The listing builds one solid part. Answer for the finished solid, in the listing's coordinates (mm). A direction names the side the tool comes from. Coordinates: 2 decimals unless noted, no trailing zeros. Write each loop counter-clockwise with the first axis right and the second up, starting at its lowest first coordinate (ties: lowest second). Pieces come first, ordered by that corner, then holes.
Autodesk Inventor part; units mm, degrees
ref_plane "YZ Plane" through (0, 0, 0) normal (1, 0, 0) x (0, 1, 0)
ref_plane "XZ Plane" through (0, 0, 0) normal (0, 1, 0) x (-1, 0, 0)
ref_plane "XY Plane" through (0, 0, 0) normal (0, 0, 1) x (1, 0, 0)
sketch "Sketch1" plane through (0, 0, 0) normal (0, 1, 0) x (-1, 0, 0)
  line L0 (4, 7.5) -> (-4, 7.5)
  line L1 (-4, 7.5) -> (-4, -7.5)
  line L2 (-4, -7.5) -> (4, -7.5)
  line L3 (4, -7.5) -> (4, 7.5)
  line L4 (4, 7.5) -> (-4, -7.5) construction
  line L5 (-4, 7.5) -> (4, -7.5) construction
  point P0 (0, 0)
  dimension "d0" = 8
  dimension "d1" = 15
extrude "Extrusion1" add sketch "Sketch1" along normal blind 10
sketch "Sketch2" plane through (0, 10, 0) normal (0, 1, 0) x (1, 0, 0)
  line L0 (4, 7.5) -> (-4, 7.5)
  line L1 (-1.5, -7.5) -> (1.5, -7.5)
  line L2 (1.5, -7.5) -> (1.5, 7.5)
  line L3 (1.5, 7.5) -> (-1.5, 7.5)
  line L4 (-1.5, 7.5) -> (-1.5, -7.5)
  line L5 (-1.5, -7.5) -> (1.5, 7.5) construction
  line L6 (1.5, -7.5) -> (-1.5, 7.5) construction
  point P0 (0, 0)
  dimension "d4" = 3
extrude "Extrusion2" cut sketch "Sketch2" against normal blind 5
thicken "Thicken1" operation add thickness 2 both sides no extend neighbours yes toward (0, 1, 0) faces at (2.3333, 10, -2.5)
thicken "Thicken2" operation add thickness 2 both sides no extend neighbours yes toward (0, 1, 0) faces at (-3.1667, 10, -2.5)
thicken "Thicken3" operation add thickness 1 both sides no extend neighbours yes toward (0, 1, 0) faces at (-3.1667, 12, -2.5)
thicken "Thicken4" operation add thickness 1 both sides no extend neighbours yes toward (0, 1, 0) faces at (3.1667, 12, 2.5)
fillet "Fillet1" radius 1 10 edges at (4, 6.5, 7.5) (4, 6.5, -7.5) (-4, 6.5, 7.5) (-4, 6.5, -7.5) (4, 13, 0) (-4, 13, 0) (2.75, 13, -7.5) (2.75, 13, 7.5) (-2.75, 13, 7.5) (-2.75, 13, -7.5)
sketch "Sketch3" plane through (0, 0, 0) normal (0, -1, 0) x (1, 0, 0)
  arc A0 (-3, 7.5) -> (-4, 6.5) centre (-3, 6.5) ccw construction
  line L0 (-4, -6.5) -> (-4, 6.5) construction
  arc A1 (-4, -6.5) -> (-3, -7.5) centre (-3, -6.5) ccw construction
  line L1 (3, -7.5) -> (-3, -7.5) construction
  arc A2 (3, -7.5) -> (4, -6.5) centre (3, -6.5) ccw construction
  line L2 (4, 6.5) -> (4, -6.5) construction
  arc A3 (4, 6.5) -> (3, 7.5) centre (3, 6.5) ccw construction
  line L3 (-3, 7.5) -> (3, 7.5) construction
  point P0 (0, 0)
  point P1 (0, 0)
hole "Hole1" at (0, 0, 0) direction (0, 1, 0) diameter 2.85 depth 5
thicken "Thicken7" operation add thickness 0.1 both sides no extend neighbours yes toward (-1, 0, 0) faces at (1.5, 7.6667, -2.1667)
thicken "Thicken8" operation add thickness 0.1 both sides no extend neighbours yes toward (1, 0, 0) faces at (-1.5, 7.6667, 2.1667)
properties part number "zoffset"
(1) Section D-D, the plane y = 3.5 is taken. Write down the section's boundary in (x, z) (3 decimals), plus the area to 3 significant figures.
(2) This flat-tipped pin is pushed along its axis until it touches: pin 1 (0.8 mm diameter, centred on x = -0.5, z = -3.5, fed in from +Y). Where does it stop, or does it pass through?
(3) Find the intervals of material crossed by probe 1 along X at (y, z) = (10.25, -1.5); probe 2 along Z at (x, y) = (0, 2.75) (3 decimals); probe 3 along Y at (x, z) = (1, -4), in increasing order.
(4) Section B-B, the plane x = 0 is taken. Write down the section's boundary in (y, z) (3 decimals).
(5) Which of the six approach directions +Z, -Z, +X, -X, +Y, -Y give full straight-line access (tool end or side, diameter ignored) to faces 5 (the cylindrical face through (-2.211, 12.699, 7.215)), 6 (the flat face through (-1.4, 9, 0))?
(6) Section A-A, the plane y = 10.25 is taken. Write down the section's boundary in (x, z).
(7) Section C-C, the plane z = 0 is taken. Write down the section's boundary in (x, y) (3 decimals).
(8) For a pull along Z with two mould halves and no side action, classify faces 1 (the cylindrical face through (3.699, 6.084, 7.215)), 2 (the flat face through (0, 4.8, -7.5)), 3 (the flat face through (2, 13, 0)), 4 (the cylindrical face through (0.87, 2.54, 1.13)) as pulls with the +Z half, pulls with the -Z half, needs draft (parallel to the pull), parting line crosses it, or undercut.
Solution:
1. outline: (-4, -6.5) arc R1 ccw to (-3, -7.5) - (3, -7.5) arc R1 ccw to (4, -6.5) - (4, 6.5) arc R1 ccw to (3, 7.5) - (-3, 7.5) arc R1 ccw to (-4, 6.5) - close; hole circle Ø2.85 at (0, 0)
1. area: 113 mm2
2. pin 1: stops at y = 5
3. probe 1: x = -4 to -1.4, 1.4 to 4
3. probe 2: z = -7.5 to -1.425, 1.425 to 7.5
3. probe 3: y = 0 to 5
4. outline: (0, -7.5) - (5, -7.5) - (5, -1.425) - (0, -1.425) - close; (0, 1.425) - (5, 1.425) - (5, 7.5) - (0, 7.5) - close
5. face 5: +Z, +X, -X, +Y
5. face 6: +Z, -Z, +Y
6. outline: (-4, -6.5) arc R1 ccw to (-3, -7.5) - (-1.4, -7.5) - (-1.4, 7.5) - (-3, 7.5) arc R1 ccw to (-4, 6.5) - close; (1.4, -7.5) - (3, -7.5) arc R1 ccw to (4, -6.5) - (4, 6.5) arc R1 ccw to (3, 7.5) - (1.4, 7.5) - close
7. outline: (-4, 0) - (-1.425, 0) - (-1.425, 5) - (-1.4, 5) - (-1.4, 13) - (-3, 13) arc R1 ccw to (-4, 12) - close; (1.4, 5) - (1.425, 5) - (1.425, 0) - (4, 0) - (4, 12) arc R1 ccw to (3, 13) - (1.4, 13) - close
8. face 1: pulls with the +Z half
8. face 2: pulls with the -Z half
8. face 3: needs draft
8. face 4: undercut
